```python
from build123d import *

# Parameters (mm, degrees)
EXTRUDE_1_OUTLINE_R   = 2.65
EXTRUDE_1_OUTLINE_R_2 = 3
EXTRUDE_1_DEPTH       = 10
CUT_EXTRUDE_1_DEPTH   = 5
FILLET_2_R            = 0.5
FILLET_3_R            = 0.5


# Read off the part's stored shape, not the designer's step: Бобышка-Вытянуть1
with BuildPart() as part:
    # Бобышка-Вытянуть1 outline → Бобышка-Вытянуть1 (new body)
    with BuildSketch(Plane(origin=(0, 0, 0), x_dir=(1, 0, 0), z_dir=(0, 1, 0))):
        with BuildLine():
            add(Edge.make_bspline(
                [(18.415201064, 16.136192912), (8.099804211, 18.278215903), (7.946140725, 9.450828153), (8.545020219, 1.48873653), (8.620156017, 0.717920777)],
                knots=[0, 0, 0, 0, 0.640184332, 0.711315924, 0.711315924, 0.711315924, 0.711315924], degree=3))
            ThreePointArc((18.415201064, 16.136192912), (28.93870742, 24.192739926), (20.02397796, 33.999866645))
            add(Edge.make_bspline(
                [(8.973177852, 49.305680737), (6.927050039, 38.283305713), (13.265956439, 34.007939827), (20.02397796, 33.999866645)],
                knots=[0, 0, 0, 0, 0.587985905, 0.587985905, 0.587985905, 0.587985905], degree=3))
            ThreePointArc((8.973177852, 49.305680737), (3.569296499, 58.26196844), (-6.656088527, 56.057762419))
            add(Edge.make_bspline(
                [(-31.086724645, 46.588079502), (-19.789574651, 43.949152129), (-13.613870041, 47.607425407), (-7.2630146, 55.254087082), (-6.656088527, 56.057762419)],
                knots=[0, 0, 0, 0, 0.709310605, 0.788122895, 0.788122895, 0.788122895, 0.788122895], degree=3))
            ThreePointArc((-31.086724645, 46.588079502), (-41.755710839, 38.490664399), (-32.559488638, 28.752856895))
            add(Edge.make_bspline(
                [(-32.559488638, 28.752856895), (-24.340075334, 29.891987935), (-11.988968241, 13.137863403), (-8.356742025, -2.233240408)],
                knots=[0, 0, 0, 0, 0.797106576, 0.797106576, 0.797106576, 0.797106576], degree=3))
            ThreePointArc((-8.356742025, -2.233240408), (1.481446867, -8.522195444), (8.620156017, 0.717920777))
        make_face()
        Circle(EXTRUDE_1_OUTLINE_R, mode=Mode.SUBTRACT)
        with Locations((19.974984355, 25)):
            Circle(EXTRUDE_1_OUTLINE_R_2, mode=Mode.SUBTRACT)
        with Locations((-32.786239492, 37.75)):
            Circle(EXTRUDE_1_OUTLINE_R_2, mode=Mode.SUBTRACT)
        Polygon((-8.349392166, 37.982099134), (4.227404243, 34.795225893), (5.082951506, 21.849183724), (-6.965087616, 17.034962885), (-15.266732554, 27.005652946), align=None, mode=Mode.SUBTRACT)
        with Locations((0, 50)):
            Circle(EXTRUDE_1_OUTLINE_R_2, mode=Mode.SUBTRACT)
    extrude(amount=EXTRUDE_1_DEPTH)

    # Эскиз2 → Вырез-Вытянуть1 (cut)
    with BuildSketch(Plane(origin=(0, 10, 0), x_dir=(1, 0, 0), z_dir=(0, 1, 0))):
        Polygon((5.030262391, 52.833689046), (0.061084495, 55.773179541), (-4.969177896, 52.939490495), (-5.030262391, 47.166310954), (-0.061084495, 44.226820459), (4.969177896, 47.060509505), align=None)
    extrude(amount=-CUT_EXTRUDE_1_DEPTH, mode=Mode.SUBTRACT)

    # Скругление2
    fillet_2_edges = [part.edges().sort_by_distance(p)[0] for p in [
        (-2.65, 0, 0),
    ]]
    fillet(fillet_2_edges, radius=FILLET_2_R)

    # Скругление3
    fillet_3_edges = [part.edges().sort_by_distance(p)[0] for p in [
        (-2.65, 10, 0),
    ]]
    fillet(fillet_3_edges, radius=FILLET_3_R)


solid = part.part
```
Geometry check sheet. Reference: the model listing, model coordinates, mm. A direction names the side the tool comes from. Coordinates: 2 decimals unless noted, no trailing zeros.
Item 1: Scan lines: line 1 along X through (y, z) = (8.25, -27); line 2 along X through (y, z) = (4, -25); line 3 along Z through (x, y) = (0, 2.5). Record each from-to range of solid material in increasing order.
Item 2: Tool access check on faces 1 (the flat face through (-14, 0, -33)), 2 (the flat face through (2.58, 7.535, -54.283)), 3 (the flat face through (4.65, 4.93, -28.41)). Record the directions out of +Z, -Z, +X, -X, +Y, -Y that give a thin tool (end or side, any length) a straight path to the whole face; none if there is none.
Item 3: Mould release check, pull along Z, two halves, no side actions. Record for faces 4 (the flat face through (-14, 10, -33)), 5 (the flat face through (-2.58, 7.535, -45.717)), 6 (the cylindrical face through (28.92, 4.93, -23.99)), 7 (the flat face through (-0.857, 4.93, -19.476)): released by +Z, released by -Z, zero draft, split by the parting line, or undercut.
Item 4: Section check A-A (z = -25). Count the separate pieces of the cut face and the enclosed holes in it, plus the area to 3 significant figures.
Item 5: Depth check by flat-ended pin: pin 1 (3 mm diameter, centred on x = -9, y = 4, fed in from +Z); pin 2 (4 mm diameter, centred on y = 3.5, z = -31.5, fed in from +X); pin 3 (4 mm diameter, centred on y = 9, z = -23.5, fed in from -X). Enter the tip coordinate at first touch or a pass-through.
Check sheet entries:
1. line 1: x = -26.49 to -15.26, 4.74 to 17.74, 22.21 to 28.75
1. line 2: x = -23.84 to -13.6, 4.87 to 16.97, 22.97 to 28.97
1. line 3: z = -59 to -53, -47 to -35.87, -19.82 to -2.65, 2.65 to 8.65
2. face 1: +Z, -Z, +X, -X, -Y
2. face 2: +Y
2. face 3: +Y, -Y
3. face 4: zero draft
3. face 5: undercut
3. face 6: split by the parting line
3. face 7: undercut
4. separate pieces: 3
4. enclosed holes: 0
4. area: 283 mm2
5. pin 1: stops at z = 4.31
5. pin 2: stops at x = 27.77
5. pin 3: stops at x = -24.43
